Design review of the part shown in the three views and the two pictorial views. Dimensions are in mm from the part's minimum x, y and z. A direction names the side the tool comes from. Coordinates: 2 decimals unless noted, no trailing zeros. Loops run counter-clockwise (first coordinate to the right, second up) from the corner with the lowest first, then second, coordinate; pieces in that order, holes last. Notation, with made-up numbers: (40.25, 75.5) -> (70.25, 75.5) arc R17 ccw to (70.25, 93.5) -> close; hole circle Ø6 at (-2.75, 53). An arc over 180 degrees is marked (long way). One line per item, written item: value. Start each with the question number.
1. Add section A-A on x = 19.5. Write out the cut boundary in (y, z).
2. Draft analysis for pull direction X (two halves, no side actions). For the marked faces 5, 6 and 7, state which applies: pulls with the +X half, pulls with the -X half, needs draft (parallel to the pull), parting line crosses it, or undercut.
3. Insertion check: pin 1 (4 mm diameter, centred on x = 3.5, y = 5, fed in from +Z); pin 2 (1.5 mm diameter, centred on y = 5.5, z = 3.5, fed in from -X); pin 3 (2 mm diameter, centred on y = 7.5, z = 1.5, fed in from -X). Each pin has a flat end and moves straight along its axis. Give the tip position at first contact, or say it passes through.
4. Machinability: for the marked faces 1, 2, 3 and 4, which of the approach directions +Z, -Z, +X, -X, +Y, -Y give a long, thin tool a straight path to every point of the face, cutting with its end or side? Answer none if there is none.
5. For probe 1 along Y at (x, z) = (19.5, 1.45); probe 2 along X at (y, z) = (5.5, 6); probe 3 along Y at (x, z) = (2.5, 1.4), list the stretches that pass through material, from the lowest coordinate up.
6. Add section B-B on z = 6. Write out the cut boundary in (x, y), plus the area to 3 significant figures.
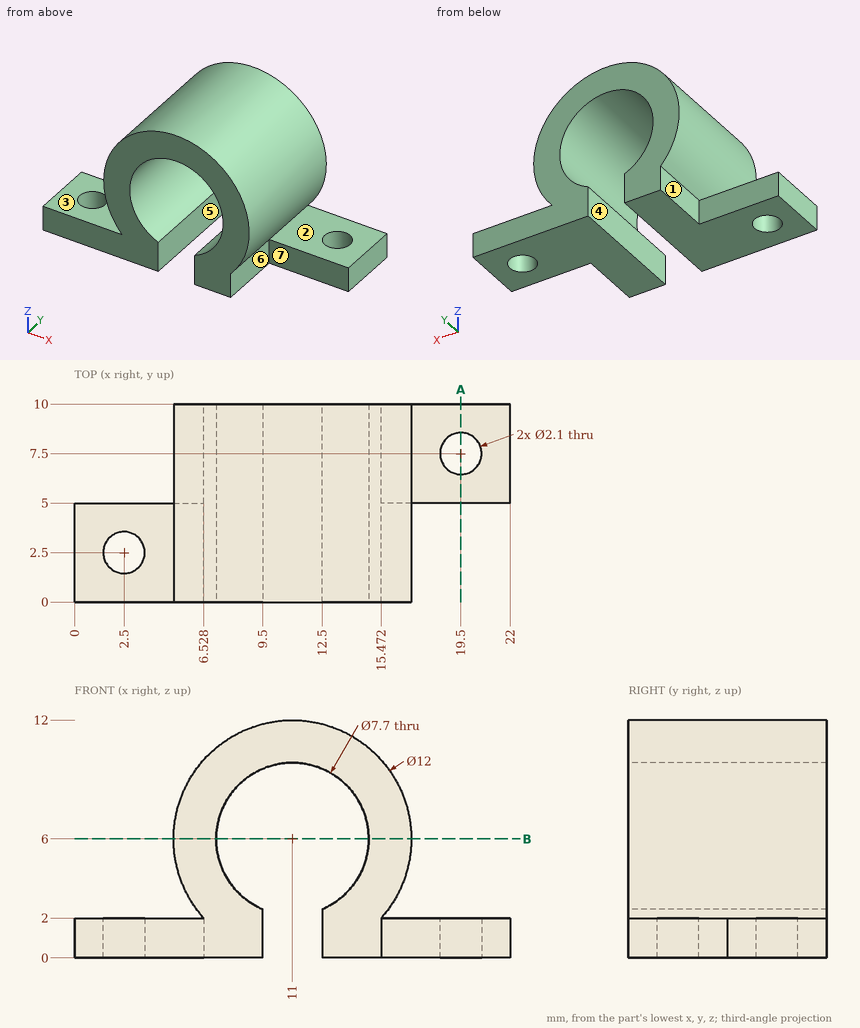
Worked answers:
1. outline: (5, 0) -> (6.45, 0) -> (6.45, 2) -> (5, 2) -> close; (8.55, 0) -> (10, 0) -> (10, 2) -> (8.55, 2) -> close
2. face 5: undercut
2. face 6: pulls with the +X half
2. face 7: needs draft
3. pin 1: stops at z = 8.4
3. pin 2: stops at x = 5.26
3. pin 3: stops at x = 6.13
4. face 1: -Z, -X, +Y
4. face 2: +X, +Y, -Y
4. face 3: -X, +Y, -Y
4. face 4: -Z, +Y, -Y
5. probe 1: y = 5 to 6.45, 8.55 to 10
5. probe 2: x = 5 to 7.15, 14.85 to 17
5. probe 3: y = 0 to 1.45, 3.55 to 5
6. outline: (5, 0) -> (7.15, 0) -> (7.15, 10) -> (5, 10) -> close; (14.85, 0) -> (17, 0) -> (17, 10) -> (14.85, 10) -> close
6. area: 43.0 mm²
